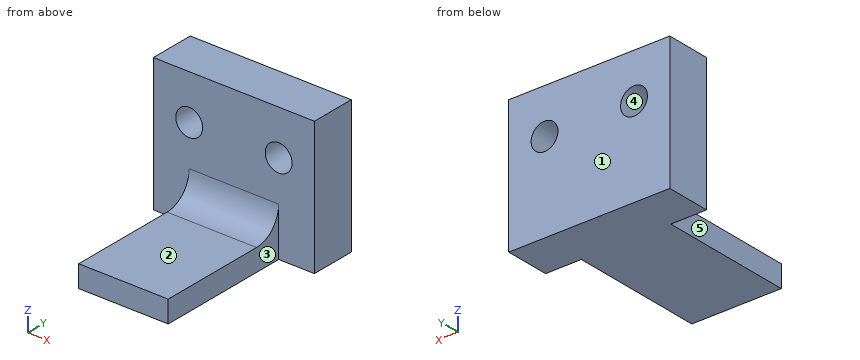
from build123d import *

# Parameters (mm, degrees)
SKETCH1_W           = 18
SKETCH1_H           = 10
SKETCH1_R           = 1.5
BOSS_EXTRUDE1_DEPTH = 5
SKETCH2_W           = 18
SKETCH2_H           = 5
BOSS_EXTRUDE2_DEPTH = 5
SKETCH3_W           = 10
SKETCH3_H           = 2.44730383
BOSS_EXTRUDE3_DEPTH = 15
BOSS_EXTRUDE5_DEPTH = 10


with BuildPart() as part:
    # Sketch1 → Boss-Extrude1 (new body)
    with BuildSketch(Plane(origin=(0, 0, 0), x_dir=(1, 0, 0), z_dir=(0, 1, 0))):
        Rectangle(SKETCH1_W, SKETCH1_H)
        with Locations(Location((-5, 0, 0), (0, 0, 270))):
            Circle(SKETCH1_R, mode=Mode.SUBTRACT)
        with Locations(Location((5, 0, 0), (0, 0, 270))):
            Circle(SKETCH1_R, mode=Mode.SUBTRACT)
    extrude(amount=BOSS_EXTRUDE1_DEPTH)

    # Sketch2 → Boss-Extrude2 (add)
    with BuildSketch(Plane(origin=(0, 0, -5), x_dir=(-1, 0, 0), z_dir=(0, 0, -1))):
        with Locations((0, 2.5)):
            Rectangle(SKETCH2_W, SKETCH2_H)
    extrude(amount=BOSS_EXTRUDE2_DEPTH)

    # Sketch3 → Boss-Extrude3 (add)
    with BuildSketch(Plane.XZ):
        with Locations((0, -8.776348085)):
            Rectangle(SKETCH3_W, SKETCH3_H)
    extrude(amount=BOSS_EXTRUDE3_DEPTH)

    # Sketch4 → Boss-Extrude5 (add)
    with BuildSketch(Plane(origin=(5, 0, 0), x_dir=(0, 0, -1), z_dir=(1, 0, 0))):
        with BuildLine():
            Line((4.55269617, 0), (7.55269617, 0))
            Line((7.55269617, 0), (7.55269617, -3))
            ThreePointArc((7.55269617, -3), (6.674016513, -0.878679656), (4.55269617, 0))
        make_face()
    extrude(amount=-BOSS_EXTRUDE5_DEPTH)


solid = part.part
For this review, take the finished solid that the model builds, in its own axes (mm). Face numbers are marked on the shaded views. A direction names the side the tool comes from. Round coordinates to 2 decimals unless told otherwise and drop trailing zeros. Loops run counter-clockwise (first coordinate to the right, second up) from the corner with the lowest first, then second, coordinate; pieces in that order, holes last. Notation, with made-up numbers: (-15, -17.75) - (16, -17.75) arc R22 ccw to (16, 21.25) - close; hole circle Ø11 at (55, 5.25). An arc over 180 degrees is marked (long way). Use one line per item in the form item = value.
Item 1: Consider section A-A on z = 0. Write out the cut boundary in (x, y).
Answers:
outline = (-9, 0) - (-6.5, 0) - (-6.5, 5) - (-9, 5) - close; (-3.5, 0) - (3.5, 0) - (3.5, 5) - (-3.5, 5) - close; (6.5, 0) - (9, 0) - (9, 5) - (6.5, 5) - close
Item 2: Clearance check with flat-ended pins moving along their axes: P1, Ø1, axis at x = 3, y = -1.5, coming from the +Z side; P2, Ø4, axis at x = -5, z = 0, coming from the +Y side; P3, Ø8, axis at x = 0.5, y = -10, coming from the +Z side; P4, Ø1, axis at x = 2.5, z = 3, coming from the -Y side. State where each tip first meets the part, or that it passes through.
Answers:
P1 = -6.79
P2 = 5
P3 = -7.55
P4 = 0
Item 3: Consider section C-C on y = 3.75. Write out the cut boundary in (x, z), then the cut area to 3 significant figures.
Answers:
outline = (-9, -10) - (9, -10) - (9, 5) - (-9, 5) - close; hole circle Ø3 at (-5, 0); hole circle Ø3 at (5, 0)
area = 256 mm^2
Item 4: Consider section B-B on x = -6.25. Write out the cut boundary in (y, z), then the cut area to 3 significant figures.
Answers:
outline = (0, -10) - (5, -10) - (5, -0.83) - (0, -0.83) - close; (0, 0.83) - (5, 0.83) - (5, 5) - (0, 5) - close
area = 66.7 mm^2
Item 5: Mouldability with a two-part tool opening along X and no side actions: class the marked faces 3, 4 and 5 as +X half, -X half, draft (parallel to the pull), parting line (faces both ways), or undercut.
Answers:
face_3 = +X half
face_4 = undercut
face_5 = -X half
Item 6: For line 1 (X direction, y = 3.4, z = 0); line 2 (Z direction, x = -1, y = -13.5); line 3 (Y direction, x = -2.5, z = 0), list the stretches that pass through material, from the lowest coordinate up.
Answers:
line_1 = -9 to -6.5, -3.5 to 3.5, 6.5 to 9
line_2 = -10 to -7.55
line_3 = 0 to 5
Item 7: Consider section D-D on x = 1.75. Write out the cut boundary in (y, z).
Answers:
outline = (-15, -10) - (5, -10) - (5, 5) - (0, 5) - (0, -4.55) arc R3 cw to (-3, -7.55) - (-15, -7.55) - close
Item 8: Tool access review of the marked faces 1 and 2: name each direction out of +Z, -Z, +X, -X, +Y, -Y from which nothing blocks a thin tool from reaching the whole face with its end or side.
Answers:
face_1 = +Z, -Z, +X, -X, +Y
face_2 = +Z, +X, -X, -Y
